Job drawing, mm, ordinate dimensions from the low corner. One solid piece. Give positions to 0.01 mm unless a question says otherwise; leave off trailing zeros. Order: outer loops, then holes, each group sorted by start corner. A loop starts at its lowest first (then second) coordinate and runs counter-clockwise, first axis right, second up.
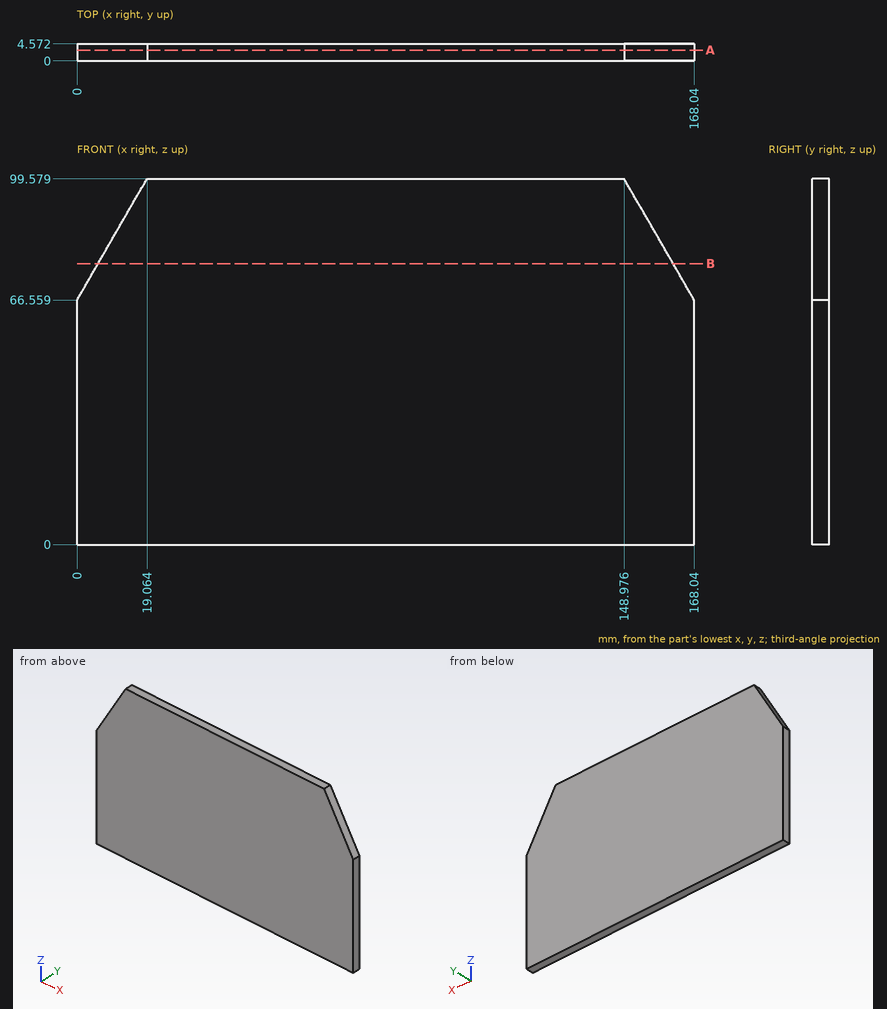
Item 1: Drop a flat-ended pin along its axis: P1, Ø1.5, axis at y = 3.5, z = 79.5, coming from the +X side. Give the stop position or say it passes through.
Item 2: Band-saw the part on B-B on z = 76.5. List the corners of the cut face in (x, y), plus the area to 3 significant figures.
Item 3: Band-saw the part on A-A on y = 2.9. List the corners of the cut face in (x, z).
Item 4: Drill centre lines: probe 1 along Z at (x, y) = (157, 3) (1 decimal); probe 2 along Z at (x, y) = (159, 2.95) (1 decimal); probe 3 along X at (y, z) = (2.5, 73). Where is each one in solid material? Low to high.
Working result:
1. P1: stops at x = 161
2. outline: (5.74, 0) - (162.3, 0) - (162.3, 4.57) - (5.74, 4.57) - close
2. area: 716 mm2
3. outline: (0, 0) - (168.04, 0) - (168.04, 66.56) - (148.98, 99.58) - (19.06, 99.58) - (0, 66.56) - close
4. probe 1: z = 0 to 85.7
4. probe 2: z = 0 to 82.2
4. probe 3: x = 3.72 to 164.32
